Work out the finished part from the listing and answer in its coordinate system (mm). A direction names the side the tool comes from. Coordinates: 2 decimals unless noted, no trailing zeros. Order: outer loops, then holes, each group sorted by start corner. A loop starts at its lowest first (then second) coordinate and runs counter-clockwise, first axis right, second up.
1. The part is cut by section D-D, the plane x = 22. Give the vertices of the cut face in (y, z).
2. Determine the mould class of faces 1 (the flat face through (-80, 7, 0)), 2 (the flat face through (-52, 7, -20)), 3 (the conical face through (-38.275, 13.347, -10.144)), 4 (the cylindrical face through (-31.8, 6.4, 9.9)) for opening direction X: +X half, -X half, draft (parallel to the pull), parting line (faces both ways), or undercut.
3. The part is cut by section C-C, the plane z = 0. Give the vertices of the cut face in (x, y).
4. Find the intervals of material crossed by probe 1 along Z at (x, y) = (-70, 7.75); probe 2 along Z at (x, y) = (-48, 1); probe 3 along Z at (x, y) = (-39.5, 2), in increasing order.
5. The part is cut by section A-A, the plane x = 50. Give the vertices of the cut face in (y, z) (3 decimals).
6. The part is cut by section B-B, the plane y = 10. Count the separate pieces of the cut face and the enclosed holes in it, then the cut area to 3 significant figures.
7. Flat-ended cylindrical pins translate along their axes: pin 1 Ø5 at (x, y) = (-52.5, 10) entering from +Z; pin 2 Ø7.5 at (x, y) = (59, 8.5) entering from -Z; pin 3 Ø6 at (x, y) = (-32.5, 7) entering from +Z; pin 4 Ø5 at (x, z) = (-50, -10) entering from -Y. Find the tip coordinate at first contact, or state that the pin passes through.
8. A tool of negligible diameter and unlimited length cuts with its end or side. For faces 5 (the cylindrical face through (67.253, 7.592, -10.121)), 6 (the flat face through (53, 7, -20)), from which of +Z, -Z, +X, -X, +Y, -Y can it reach the whole face along a straight path? Write none if from no direction.
```python
from build123d import *
from OCP.BRepFilletAPI import BRepFilletAPI_MakeChamfer

# Parameters (mm, degrees)
BOSS_EXTRUDE1_DEPTH = 15
CUT_EXTRUDE3_REACH  = 92.692
SKETCH4_R           = 30.5
SKETCH3_R           = 32.6
CUT_EXTRUDE4_DEPTH  = 7
FILLET1_R           = 10
HOLE1_D             = 6.4
HOLE1_CBORE_D       = 7.3
HOLE1_CBORE_DEPTH   = 2
CHAMFER1_SIZE       = 0.45
CHAMFER1_SIZE_2     = 2


# Read off the part's stored shape, not the designer's step: M5 Clearance Hole1
with BuildPart() as part:
    # Sketch1 → Boss-Extrude1 (new body)
    with BuildSketch(Plane(origin=(0, 0, 0), x_dir=(1, 0, 0), z_dir=(0, 1, 0))):
        with BuildLine():
            ThreePointArc((34.641016151, 20), (0, 40), (-34.641016151, 20))
            Line((-34.641016151, 20), (34.641016151, 20))
        make_face()
        with BuildLine():
            Line((34.641016151, 20), (-34.641016151, 20))
            ThreePointArc((-34.641016151, 20), (-40, 0), (-34.641016151, -20))
            Line((-34.641016151, -20), (34.641016151, -20))
            ThreePointArc((34.641016151, -20), (38.637033052, -10.352761804), (40, 0))
            ThreePointArc((40, 0), (38.637033052, 10.352761804), (34.641016151, 20))
        make_face()
        with BuildLine():
            Line((-34.641016151, 20), (-80, 20))
            Line((-80, 20), (-80, -20))
            Line((-80, -20), (-34.641016151, -20))
            ThreePointArc((-34.641016151, -20), (-40, 0), (-34.641016151, 20))
        make_face()
        with BuildLine():
            Line((80, 20), (34.641016151, 20))
            ThreePointArc((34.641016151, 20), (38.637033052, 10.352761804), (40, 0))
            ThreePointArc((40, 0), (38.637033052, -10.352761804), (34.641016151, -20))
            Line((34.641016151, -20), (80, -20))
            Line((80, -20), (80, 20))
        make_face()
        with BuildLine():
            Line((34.641016151, -20), (-34.641016151, -20))
            ThreePointArc((-34.641016151, -20), (0, -40), (34.641016151, -20))
        make_face()
    extrude(amount=BOSS_EXTRUDE1_DEPTH)

    # Sketch4 → Cut-Extrude3 (cut, up to next)
    with BuildSketch(Plane(origin=(0, 15, 0), x_dir=(1, 0, 0), z_dir=(0, 1, 0)), mode=Mode.PRIVATE) as cut_extrude3_sk1:
        with Locations(Location((0, 0, 0), (0, 0, 270))):
            Circle(SKETCH4_R)
    cut_extrude3_tool1 = extrude(cut_extrude3_sk1.sketch, amount=-CUT_EXTRUDE3_REACH, mode=Mode.PRIVATE) & part.part
    add(cut_extrude3_tool1.solids().sort_by_distance((0, 15, 0))[0], mode=Mode.SUBTRACT)

    # Sketch3 → Cut-Extrude4 (cut)
    with BuildSketch(Plane.XZ):
        with Locations(Location((0, 0, 0), (0, 0, 270))):
            Circle(SKETCH3_R)
    extrude(amount=-CUT_EXTRUDE4_DEPTH, mode=Mode.SUBTRACT)

    # M5 Clearance Hole1 outline → M5 Clearance Hole1 (revolve, cut)
    with BuildSketch(Plane(origin=(70, 0, -10), x_dir=(1, 0, 0), z_dir=(0, 0, 1))):
        Polygon((0, 0), (2.75, 0), (2.75, 14.975), (2.775, 15), (0, 15), align=None)
    revolve(axis=Axis((70, 0, -10), (0, 1, 0)), mode=Mode.SUBTRACT)

    # M5 Clearance Hole1 2 outline → M5 Clearance Hole1 2 (revolve, cut)
    with BuildSketch(Plane(origin=(50, 0, 10), x_dir=(1, 0, 0), z_dir=(0, 0, 1))):
        Polygon((0, 0), (2.75, 0), (2.75, 14.975), (2.775, 15), (0, 15), align=None)
    revolve(axis=Axis((50, 0, 10), (0, 1, 0)), mode=Mode.SUBTRACT)

    # M5 Clearance Hole1 3 outline → M5 Clearance Hole1 3 (revolve, cut)
    with BuildSketch(Plane(origin=(70, 0, 10), x_dir=(1, 0, 0), z_dir=(0, 0, 1))):
        Polygon((0, 0), (2.75, 0), (2.75, 14.975), (2.775, 15), (0, 15), align=None)
    revolve(axis=Axis((70, 0, 10), (0, 1, 0)), mode=Mode.SUBTRACT)

    # M5 Clearance Hole1 4 outline → M5 Clearance Hole1 4 (revolve, cut)
    with BuildSketch(Plane(origin=(50, 0, -10), x_dir=(1, 0, 0), z_dir=(0, 0, 1))):
        Polygon((0, 0), (2.75, 0), (2.75, 14.975), (2.775, 15), (0, 15), align=None)
    revolve(axis=Axis((50, 0, -10), (0, 1, 0)), mode=Mode.SUBTRACT)

    # M5 Clearance Hole1 5 outline → M5 Clearance Hole1 5 (revolve, cut)
    with BuildSketch(Plane(origin=(-50, 0, -10), x_dir=(1, 0, 0), z_dir=(0, 0, 1))):
        Polygon((0, 0), (2.75, 0), (2.75, 14.975), (2.775, 15), (0, 15), align=None)
    revolve(axis=Axis((-50, 0, -10), (0, 1, 0)), mode=Mode.SUBTRACT)

    # M5 Clearance Hole1 6 outline → M5 Clearance Hole1 6 (revolve, cut)
    with BuildSketch(Plane(origin=(-70, 0, 10), x_dir=(1, 0, 0), z_dir=(0, 0, 1))):
        Polygon((0, 0), (2.75, 0), (2.75, 14.975), (2.775, 15), (0, 15), align=None)
    revolve(axis=Axis((-70, 0, 10), (0, 1, 0)), mode=Mode.SUBTRACT)

    # M5 Clearance Hole1 7 outline → M5 Clearance Hole1 7 (revolve, cut)
    with BuildSketch(Plane(origin=(-50, 0, 10), x_dir=(1, 0, 0), z_dir=(0, 0, 1))):
        Polygon((0, 0), (2.75, 0), (2.75, 14.975), (2.775, 15), (0, 15), align=None)
    revolve(axis=Axis((-50, 0, 10), (0, 1, 0)), mode=Mode.SUBTRACT)

    # M5 Clearance Hole1 8 outline → M5 Clearance Hole1 8 (revolve, cut)
    with BuildSketch(Plane(origin=(-70, 0, -10), x_dir=(1, 0, 0), z_dir=(0, 0, 1))):
        Polygon((0, 0), (2.75, 0), (2.75, 14.975), (2.775, 15), (0, 15), align=None)
    revolve(axis=Axis((-70, 0, -10), (0, 1, 0)), mode=Mode.SUBTRACT)

    # Fillet1
    fillet1_edges = [part.edges().sort_by_distance(p)[0] for p in [
        (80, 7.5, -20),
        (80, 7.5, 20),
        (-80, 7.5, 20),
        (-80, 7.5, -20),
    ]]
    fillet(fillet1_edges, radius=FILLET1_R)

    # Hole1 (through all)
    with Locations(Plane(origin=(0, 15, 0), x_dir=(1, 0, 0), z_dir=(0, 1, 0))):
        with Locations((35, -10), (-35, 10), (-35, -10), (35, 10)):
            CounterBoreHole(HOLE1_D / 2, HOLE1_CBORE_D / 2, HOLE1_CBORE_DEPTH)

    # Chamfer1
    chamfer1_edges_1 = [part.edges().sort_by_distance(p)[0] for p in [
        (31.35, 13, 10),
    ]]
    chamfer1_side_1 = [part.faces().sort_by_distance(p)[0] for p in [
        (31.359, 13, 10),
    ]]
    chamfer1_edges_2 = [part.edges().sort_by_distance(p)[0] for p in [
        (31.35, 13, -10),
    ]]
    chamfer1_side_2 = [part.faces().sort_by_distance(p)[0] for p in [
        (31.359, 13, -10),
    ]]
    chamfer1_edges_3 = [part.edges().sort_by_distance(p)[0] for p in [
        (-38.65, 13, 10),
    ]]
    chamfer1_side_3 = [part.faces().sort_by_distance(p)[0] for p in [
        (-38.641, 13, 10),
    ]]
    chamfer1_edges_4 = [part.edges().sort_by_distance(p)[0] for p in [
        (-38.65, 13, -10),
    ]]
    chamfer1_side_4 = [part.faces().sort_by_distance(p)[0] for p in [
        (-38.641, 13, -10),
    ]]
    chamfer1 = BRepFilletAPI_MakeChamfer(part.part.solid().wrapped)
    for e in chamfer1_edges_1:
        chamfer1.Add(CHAMFER1_SIZE - 0.0001, CHAMFER1_SIZE_2 - 0.0001, e.wrapped, chamfer1_side_1[0].wrapped)
    for e in chamfer1_edges_2:
        chamfer1.Add(CHAMFER1_SIZE - 0.0001, CHAMFER1_SIZE_2 - 0.0001, e.wrapped, chamfer1_side_2[0].wrapped)
    for e in chamfer1_edges_3:
        chamfer1.Add(CHAMFER1_SIZE - 0.0001, CHAMFER1_SIZE_2 - 0.0001, e.wrapped, chamfer1_side_3[0].wrapped)
    for e in chamfer1_edges_4:
        chamfer1.Add(CHAMFER1_SIZE - 0.0001, CHAMFER1_SIZE_2 - 0.0001, e.wrapped, chamfer1_side_4[0].wrapped)
    add(Compound.cast(chamfer1.Shape()), mode=Mode.REPLACE)  # a hair under: the kernel refuses the full size


solid = part.part
```
Geometry says:
1. outline: (0, -33.41) - (15, -33.41) - (15, -21.12) - (7, -21.12) - (7, -24.06) - (0, -24.06) - close; (0, 24.06) - (7, 24.06) - (7, 21.12) - (15, 21.12) - (15, 33.41) - (0, 33.41) - close
2. face 1: -X half
2. face 2: draft
2. face 3: undercut
2. face 4: undercut
3. outline: (-80, 0) - (-32.6, 0) - (-32.6, 7) - (-30.5, 7) - (-30.5, 15) - (-80, 15) - close; (30.5, 7) - (32.6, 7) - (32.6, 0) - (80, 0) - (80, 15) - (30.5, 15) - close
4. probe 1: z = -20 to -12.75, -7.25 to 7.25, 12.75 to 20
4. probe 2: z = -20 to -11.89, -8.11 to 8.11, 11.89 to 20
4. probe 3: z = -20 to 20
5. outline: (0, -20) - (15, -20) - (15, -12.775) - (14.975, -12.75) - (0, -12.75) - close; (0, -7.25) - (14.975, -7.25) - (15, -7.225) - (15, 7.225) - (14.975, 7.25) - (0, 7.25) - close; (0, 12.75) - (14.975, 12.75) - (15, 12.775) - (15, 20) - (0, 20) - close
6. separate pieces: 1
6. enclosed holes: 13
6. area: 5,040 mm2
7. pin 1: stops at z = 20
7. pin 2: stops at z = -20
7. pin 3: stops at z = 27.01
7. pin 4: passes through
8. face 5: +Y, -Y
8. face 6: -Z, +X, +Y, -Y
